The listing builds one solid part. Answer for the finished solid, in the listing's coordinates (mm). Face numbers are marked on the shaded views. A direction names the side the tool comes from. Coordinates: 2 decimals unless noted, no trailing zeros. Loops run counter-clockwise (first coordinate to the right, second up) from the corner with the lowest first, then second, coordinate; pieces in that order, holes last. Notation, with made-up numbers: M 77,80 L 129,80 A13 cw 129,95 Z; hole C 53.5,67.25 d9. An arc over 180 degrees is marked long. Return JSON: item names as keys, results as strings. Group by question number.
1. Straight lines are drawn through the part: L1, parallel to X at y = 30, z = 0 (3 decimals); L2, parallel to X at y = 21, z = 3; L3, parallel to X at y = 23, z = 19.5. For each, find the intervals that lie inside material, in ascending order. Write a range as from..to.
2. Given P1, Ø5, axis at x = -69, y = 41, coming from the +Z side; P2, Ø2, axis at x = -81.33, y = 12.6, coming from the +Z side; P3, Ø1, axis at y = 13.5, z = -46, coming from the +X side; P4, Ø14.5, axis at x = 0, z = 0, coming from the -Y side, each flat-ended and moving along its own axis, determine where each tip first touches the part or whether it passes through.
3. The mould has two halves that part along X. Classify the marked faces 1, 2 and 3: pulls with the +X half, pulls with the -X half, needs draft (parallel to the pull), parting line crosses it, or undercut.
4. Section C-C (z = -10) is taken. Write down the section's boundary in (x, y).
5. Which of the six approach directions +Z, -Z, +X, -X, +Y, -Y give full straight-line access (tool end or side, diameter ignored) to the marked faces 4, 5 and 6?
6. Section B-B (y = 18) is taken. Write down the section's boundary in (x, z) (3 decimals), then the cut area to 3 significant figures.
7. Section A-A (x = 0) is taken. Write down the section's boundary in (y, z) (3 decimals).
8. Section D-D (y = 47) is taken. Write down the section's boundary in (x, z) (3 decimals).
```python
from build123d import *

# Parameters (mm, degrees)
ESQUISSE1_R             = 3.675
BOSS_EXTRU_1_DEPTH      = 60
ESQUISSE2_W             = 50
ESQUISSE2_H             = 29
ENL_V_MAT_EXTRU_1_DEPTH = 40
D_GAGEMENT_M21_D        = 2.6
D_GAGEMENT_M21_DEPTH    = 3.5
ESQUISSE4_R             = 6.35
ENL_V_MAT_EXTRU_2_DEPTH = 4
ENL_V_START             = -4
ESQUISSE5_R             = 6.35
ENL_V_MAT_EXTRU_3_DEPTH = 4
ESQUISSE6_R             = 6.35
ENL_V_MAT_EXTRU_4_DEPTH = 4


with BuildPart() as part:
    # Esquisse1 → Boss.-Extru.1 (new body)
    with BuildSketch(Plane(origin=(0, 0, 0), x_dir=(1, 0, 0), z_dir=(0, 1, 0))):
        with BuildLine():
            ThreePointArc((-98.54472285, 18), (-103.33, -13.21472285), (-72.11527715, -18))
            Line((-72.11527715, -18), (-65.055745327, -18))
            ThreePointArc((-65.055745327, -18), (66.254971265, -12.904603158), (-53.54472285, 41.100032298))
            Line((-53.54472285, 41.100032298), (-53.54472285, 18))
            Line((-53.54472285, 18), (-98.54472285, 18))
        make_face()
        with Locations(Location((-85.33, 0, 0), (0, 0, 270))):
            Circle(ESQUISSE1_R, mode=Mode.SUBTRACT)
        with Locations(Location((0, 0, 0), (0, 0, 270))):
            Circle(ESQUISSE1_R, mode=Mode.SUBTRACT)
    extrude(amount=BOSS_EXTRU_1_DEPTH)

    # Esquisse2 → Enlèv. mat.-Extru.1 (cut)
    with BuildSketch(Plane.XZ):
        with Locations((-71.58, 0)):
            Rectangle(ESQUISSE2_W, ESQUISSE2_H)
    extrude(amount=-ENL_V_MAT_EXTRU_1_DEPTH, mode=Mode.SUBTRACT)

    # Dégagement M21
    with Locations(Plane(origin=(-57.33, 24.6, -18), x_dir=(-1, 0, 0), z_dir=(0, 0, -1))):
        with Locations((0, 0), (24, 0), (24, -12), (0, -12)):
            Hole(D_GAGEMENT_M21_D / 2, depth=D_GAGEMENT_M21_DEPTH)

    # Esquisse4 → Enlèv. mat.-Extru.2 (cut)
    with BuildSketch(Plane.XZ):
        with Locations(Location((0, 0, 0), (0, 0, 270))):
            Circle(ESQUISSE4_R)
    extrude(amount=-ENL_V_MAT_EXTRU_2_DEPTH, mode=Mode.SUBTRACT)

    # Esquisse5 → Enlèv. mat.-Extru.3 (cut)
    with BuildSketch(Plane(origin=(0, 60, 0), x_dir=(1, 0, 0), z_dir=(0, 1, 0)).offset(ENL_V_START)):
        with Locations(Location((0, 0, 0), (0, 0, 90))):
            Circle(ESQUISSE5_R)
    extrude(amount=ENL_V_MAT_EXTRU_3_DEPTH, mode=Mode.SUBTRACT)

    # Esquisse6 → Enlèv. mat.-Extru.4 (cut)
    with BuildSketch(Plane(origin=(0, 60, 0), x_dir=(1, 0, 0), z_dir=(0, 1, 0))):
        with Locations(Location((-85.33, 0, 0), (0, 0, 270))):
            Circle(ESQUISSE6_R)
    extrude(amount=-ENL_V_MAT_EXTRU_4_DEPTH, mode=Mode.SUBTRACT)


solid = part.part
```
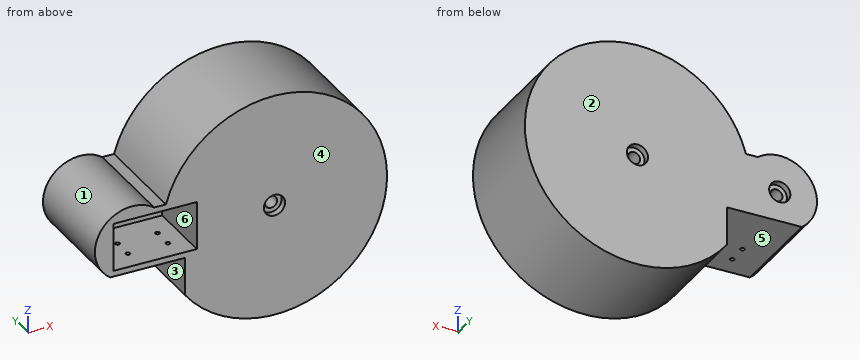
Worked out:
{
 "1": {"L1": "-107.66..-96.58, -46.58..-3.675, 3.675..67.5", "L2": "-107.46..-96.58, -46.58..-2.12, 2.12..67.43", "L3": "-96.21..-74.45, -64.62..64.62"},
 "2": {"P1": "z = 18", "P2": "z = 22.13", "P3": "x = 49.86", "P4": "y = 0"},
 "3": {"face 1": "undercut", "face 2": "needs draft", "face 3": "pulls with the -X half"},
 "4": {"outline": "M -105.3,0 L -96.58,0 L -96.58,40 L -46.58,40 L -46.58,0 L 66.76,0 L 66.76,60 L -105.3,60 Z"},
 "5": {"face 4": "+Z, -Z, +X, -X, -Y", "face 5": "-Z, -X, +Y, -Y", "face 6": "-Y"},
 "6": {"outline": "M -98.545,-18 L -53.545,-18 L -53.545,-41.1 A67.5 ccw long -65.056,18 L -72.115,18 A22.33 ccw Z; hole M -96.58,-14.5 L -46.58,-14.5 L -46.58,14.5 L -96.58,14.5 Z; hole C 0,0 d7.35", "area": "14,100 mm^2"},
 "7": {"outline": "M 0,-67.5 L 60,-67.5 L 60,-6.35 L 56,-6.35 L 56,-3.675 L 4,-3.675 L 4,-6.35 L 0,-6.35 Z; M 0,6.35 L 4,6.35 L 4,3.675 L 56,3.675 L 56,6.35 L 60,6.35 L 60,67.5 L 0,67.5 Z"},
 "8": {"outline": "M -98.545,-18 L -53.545,-18 L -53.545,-41.1 A67.5 ccw long -65.056,18 L -72.115,18 A22.33 ccw Z; hole C -85.33,0 d7.35; hole C 0,0 d7.35"}
}
